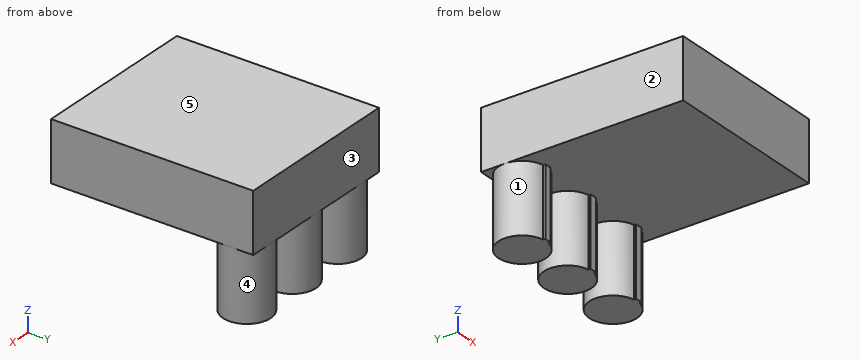
```python
from build123d import *

# Parameters (mm, degrees)
SKETCH1_R                = 11.20775
BOSS_EXTRUDE1_DEPTH      = 60.325
LPATTERN1_COUNT          = 2
LPATTERN1_PITCH          = 29.21
LPATTERN1_2_COUNT        = 2
LPATTERN1_2_PITCH        = 29.21
SKETCH2_W                = 80.8355
SKETCH2_H                = 27.94
BOSS_EXTRUDE2_DEPTH      = 11.20775
BOSS_EXTRUDE2_DEPTH_BACK = 84.04225


with BuildPart() as part:
    # Sketch1 → Boss-Extrude1 (new body)
    with BuildSketch(Plane.XY):
        Circle(SKETCH1_R)
        with BuildLine():
            ThreePointArc((1.7145, -11.075836303), (0, -11.20775), (-1.7145, -11.075836303))
            Line((-1.7145, -11.075836303), (-1.7145, -12.104536303))
            Line((-1.7145, -12.104536303), (1.7145, -12.104536303))
            Line((1.7145, -12.104536303), (1.7145, -11.075836303))
        make_face()
    extrude(amount=BOSS_EXTRUDE1_DEPTH)


with BuildPart() as lpattern1_1:
    # LPattern1: pattern copy
    add(part.part.moved(Location(Vector(1, 0, 0) * (1 * LPATTERN1_PITCH))))


with BuildPart() as lpattern1_2_1:
    # LPattern1 2: pattern copy
    add(part.part.moved(Location(Vector(-1, 0, 0) * (1 * LPATTERN1_2_PITCH))))


with BuildPart() as lpattern1_2_2:
    # LPattern1 2: pattern copy
    add(lpattern1_1.part.moved(Location(Vector(-1, 0, 0) * (1 * LPATTERN1_2_PITCH))))


with BuildPart() as part_1:
    add(part.part)

    add(lpattern1_1.part)  # Boss-Extrude2 merges LPattern1_1

    add(lpattern1_2_1.part)  # Boss-Extrude2 merges LPattern1 2_1

    add(lpattern1_2_2.part)  # Boss-Extrude2 merges LPattern1 2_2
    # Sketch2 → Boss-Extrude2 (add, two sides)
    with BuildSketch(Plane(origin=(0, 0, 0), x_dir=(1, 0, 0), z_dir=(0, 1, 0))) as boss_extrude2_sk:
        with Locations((0, -46.355)):
            Rectangle(SKETCH2_W, SKETCH2_H)
    extrude(amount=BOSS_EXTRUDE2_DEPTH)
    extrude(boss_extrude2_sk.sketch, amount=-BOSS_EXTRUDE2_DEPTH_BACK)


solid = part_1.part
```
Geometry: final body of the model. Coordinates: model frame, mm. Face numbers are marked on the shaded views. A direction names the side the tool comes from. Round coordinates to 2 decimals unless told otherwise and drop trailing zeros. Order: outer loops, then holes, each group sorted by start corner. A loop starts at its lowest first (then second) coordinate and runs counter-clockwise, first axis right, second up. Notation, with made-up numbers: M 60.25,60.5 L 104.25,60.5 A24 cw 104.25,91.5 Z; hole C 80,22.25 d7. An arc over 180 degrees is marked long. One line per item, written item: value.
(1) Cut plane B-B (y = -8). Return the cut outline in (x, z) (3 decimals), and give its area (3 significant figures).
Result sheet:
outline: M -40.418,32.385 L -37.059,32.385 L -37.059,0 L -21.361,0 L -21.361,32.385 L -7.849,32.385 L -7.849,0 L 7.849,0 L 7.849,32.385 L 21.361,32.385 L 21.361,0 L 37.059,0 L 37.059,32.385 L 40.418,32.385 L 40.418,60.325 L -40.418,60.325 Z
area: 3,780 mm2
(2) Cut plane C-C (y = -73). Return the cut outline in (x, z) (3 decimals), and give its area (3 significant figures).
Result sheet:
outline: M -40.418,32.385 L 40.418,32.385 L 40.418,60.325 L -40.418,60.325 Z
area: 2,260 mm2
(3) Cut plane A-A (z = 28.5). Return the cut outline in (x, y), and give its area (3 significant figures).
Result sheet:
outline: M -30.92,-12.1 L -27.5,-12.1 L -27.5,-11.08 A11.21 ccw long -30.92,-11.08 Z; M -1.71,-12.1 L 1.71,-12.1 L 1.71,-11.08 A11.21 ccw long -1.71,-11.08 Z; M 27.5,-12.1 L 30.92,-12.1 L 30.92,-11.08 A11.21 ccw long 27.5,-11.08 Z
area: 1,190 mm2
(4) Pull-direction query (X, two-part tool) for the marked faces 1, 2 and 3; classes: pulls with the +X half, pulls with the -X half, needs draft (parallel to the pull), parting line crosses it, or undercut.
Result sheet:
face 1: undercut
face 2: pulls with the -X half
face 3: needs draft
(5) Line query: probe 1 along Z at (x, y) = (31.5, -17.5) (3 decimals); probe 2 along Y at (x, z) = (-5, 3); probe 3 along Y at (x, z) = (-34.5, 2). Output: solid intervals per line, ascending. Write a range as [from, to].
Result sheet:
probe 1: [32.385, 60.325]
probe 2: [-10.03, 10.03]
probe 3: [-9.88, 9.88]
(6) Pin query (flat end, axial travel): P1, Ø0.5, axis at y = -11.5, z = 13, coming from the +X side; P2, Ø0.5, axis at y = -11.5, z = 10, coming from the -X side; P3, Ø4, axis at x = -0.5, z = 18.5, coming from the -Y side. Return the tip coordinate at first contact, or that it passes through.
Result sheet:
P1: x = 30.92
P2: x = -30.92
P3: y = -12.1
(7) Reachability of the marked faces 4 and 5 from +Z, -Z, +X, -X, +Y, -Y: full face, straight path, thin tool, end or side. Return the list, or none.
Result sheet:
face 4: -Z
face 5: +Z, +X, -X, +Y, -Y
